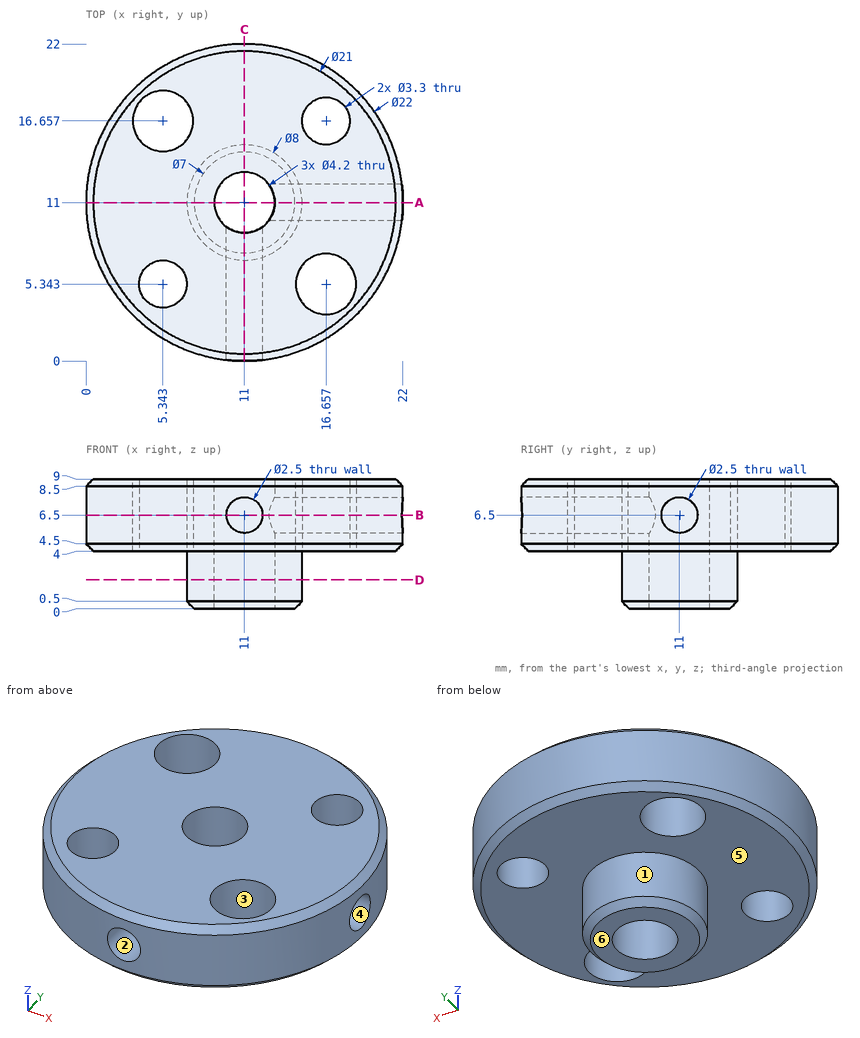
Design review of the part shown in the three views and the two pictorial views. Dimensions are in mm from the part's minimum x, y and z. A direction names the side the tool comes from. Give positions to 0.01 mm unless a question says otherwise; leave off trailing zeros. Loops run counter-clockwise (first coordinate to the right, second up) from the corner with the lowest first, then second, coordinate; pieces in that order, holes last. Notation, with made-up numbers: (70.5, -5) - (84.5, -5) arc R26 ccw to (84.5, 32) - close; hole circle Ø7 at (68.5, 61). An arc over 180 degrees is marked (long way). Use CSV: the item, a comma, the result in double quotes. Start each with the question number.
1. Wall thickness on L1, parallel to X at y = 6.5, z = 8.25 (1 decimal); L2, parallel to X at y = 4.5, z = 8 (1 decimal); L3, parallel to Y at x = 16, z = 6.5: over which ranges is each line inside the solid? List them lowest first.
2. Insertion check: P1, Ø4, axis at y = 6.5, z = 4, coming from the -X side; P2, Ø1.5, axis at y = 8, z = 1.5, coming from the -X side; P3, Ø2, axis at y = 15.5, z = 3.5, coming from the -X side. Each pin has a flat end and moves straight along its axis. Give the tip position at first contact, or say it passes through.
3. Add section C-C (x = 11). State the section outline as (y, z) points, plus the area to 3 significant figures.
4. Machinability: for the marked faces 4, 5 and 6, which of the approach directions +Z, -Z, +X, -X, +Y, -Y give a long, thin tool a straight path to every point of the face, cutting with its end or side? Answer none if there is none.
5. Draft analysis for pull direction Y (two halves, no side actions). For the marked faces 1, 2 and 3, state which applies: released by +Y, released by -Y, zero draft, split by the parting line, or undercut.
6. Add section A-A (y = 11). State the section outline as (x, z) points, plus the area to 3 significant figures.
7. Add section B-B (z = 6.5). State the section outline as (x, y) points, plus the area to 3 significant figures.
8. Add section D-D (z = 2). State the section outline as (x, y) points, plus the area to 3 significant figures.
Results found:
1,L1,"x = 1 to 4.2, 6.5 to 14.9, 18.4 to 21"
1,L2,"x = 2.1 to 3.9, 6.8 to 14.7, 18.6 to 19.9"
1,L3,"y = 1.2 to 3.35, 7.34 to 9.75, 12.25 to 15.14, 18.17 to 20.8"
2,P1,"stops at x = 0.3"
2,P2,"stops at x = 7.69"
2,P3,"stops at x = 0.88"
3,outline,"(0, 4.5) - (0.5, 4) - (7, 4) - (7, 0.5) - (7.5, 0) - (8.9, 0) - (8.9, 5.25) - (0, 5.25) - close; (0, 7.75) - (8.9, 7.75) - (8.9, 9) - (0.5, 9) - (0, 8.5) - close; (13.1, 0) - (14.5, 0) - (15, 0.5) - (15, 4) - (21.5, 4) - (22, 4.5) - (22, 8.5) - (21.5, 9) - (13.1, 9) - close"
3,area,"81.2 mm²"
4,face 4,"+X"
4,face 5,"-Z"
4,face 6,"-Z, +X, -X, +Y, -Y"
5,face 1,"split by the parting line"
5,face 2,"zero draft"
5,face 3,"undercut"
6,outline,"(0, 4.5) - (0.5, 4) - (7, 4) - (7, 0.5) - (7.5, 0) - (8.9, 0) - (8.9, 9) - (0.5, 9) - (0, 8.5) - close; (13.1, 0) - (14.5, 0) - (15, 0.5) - (15, 4) - (21.5, 4) - (22, 4.5) - (22, 5.25) - (13.1, 5.25) - close; (13.1, 7.75) - (22, 7.75) - (22, 8.5) - (21.5, 9) - (13.1, 9) - close"
6,area,"81.2 mm²"
7,outline,"(9.75, 0.07) - (9.75, 9.31) arc R2.1 cw (long way) to (12.69, 12.25) - (21.93, 12.25) arc R11 ccw (long way) to start; (12.25, 0.07) arc R11 ccw to (21.93, 9.75) - (12.69, 9.75) arc R2.1 cw to (12.25, 9.31) - close; hole circle Ø4.2 at (5.34, 16.66); hole circle Ø3.3 at (5.34, 5.34); hole circle Ø4.2 at (16.66, 5.34); hole circle Ø3.3 at (16.66, 16.66)"
7,area,"276 mm²"
8,outline,"circle Ø8 at (11, 11); hole circle Ø4.2 at (11, 11)"
8,area,"36.4 mm²"
